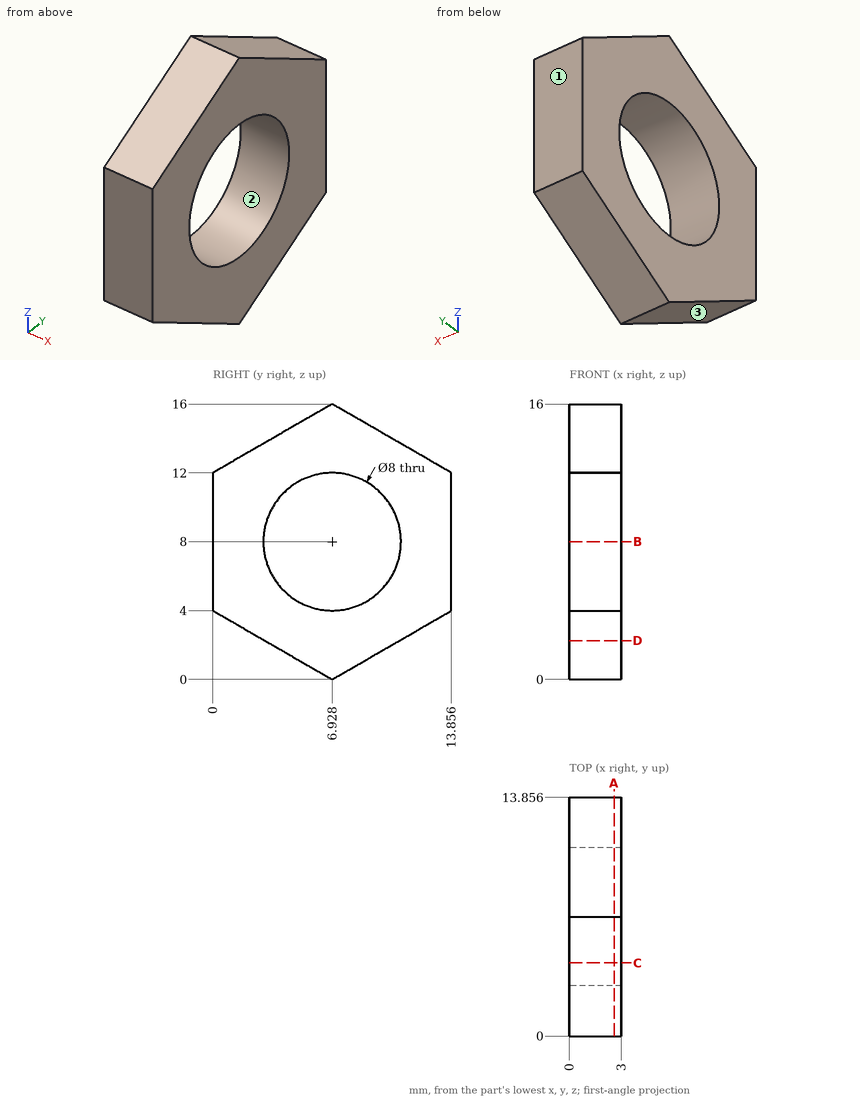
Here's the drawing with two shaded views (mm, measured from the low corner). I have some questions. Coordinates: 2 decimals unless noted, no trailing zeros. Loops run counter-clockwise (first coordinate to the right, second up) from the corner with the lowest first, then second, coordinate; pieces in that order, holes last. Notation, with made-up numbers: M 9,39.25 L 66,39.25 A14 cw 66,55.25 Z; hole C 66.25,87 d7. An arc over 180 degrees is marked long. Put each result on its own line as item: value. Start each with the question number.
(1) Imagine slicing it at B-B on z = 8. List the corners of the cut face in (x, y) for me.
(2) Imagine slicing it at C-C on y = 4.25. List the corners of the cut face in (x, z) for me.
(3) Imagine slicing it at A-A on x = 2.6. List the corners of the cut face in (y, z) for me.
(4) I need wall thicknesses on probe 1 along Y at (x, z) = (1.7, 8); probe 2 along Z at (x, y) = (1.2, 3.5); probe 3 along Z at (x, y) = (2.2, 10) (1 decimal). Which ranges of each line are inside material? Lowest first, please.
(5) Imagine slicing it at D-D on z = 2.25. List the corners of the cut face in (x, y) for me (1 decimal).
(6) Will this pin go through, and if not, where does the flat tip stop? pin 1 Ø4 at (y, z) = (2, 5.5) entering from -X.
(7) We'd pull the mould along Z, two halves only. Please class the marked faces 1, 2 and 3: +Z half, -Z half, draft (parallel to the pull), parting line (faces both ways), or undercut.
Worked answers:
1. outline: M 0,0 L 3,0 L 3,2.93 L 0,2.93 Z; M 0,10.93 L 3,10.93 L 3,13.86 L 0,13.86 Z
2. outline: M 0,1.55 L 3,1.55 L 3,5.03 L 0,5.03 Z; M 0,10.97 L 3,10.97 L 3,14.45 L 0,14.45 Z
3. outline: M 0,4 L 6.93,0 L 13.86,4 L 13.86,12 L 6.93,16 L 0,12 Z; hole C 6.93,8 d8
4. probe 1: y = 0 to 2.93, 10.93 to 13.86
4. probe 2: z = 1.98 to 5.94, 10.06 to 14.02
4. probe 3: z = 1.8 to 5.4, 10.6 to 14.2
5. outline: M 0,3 L 3,3 L 3,10.8 L 0,10.8 Z
6. pin 1: stops at x = 0
7. face 1: draft
7. face 2: undercut
7. face 3: -Z half
